Autodesk Inventor part; units mm, degrees
ref_plane "YZ Plane" through (0, 0, 0) normal (1, 0, 0) x (0, 1, 0)
ref_plane "XZ Plane" through (0, 0, 0) normal (0, 1, 0) x (-1, 0, 0)
ref_plane "XY Plane" through (0, 0, 0) normal (0, 0, 1) x (1, 0, 0)
sketch "Эскиз1" plane through (0, 0, 0) normal (0, 1, 0) x (-1, 0, 0)
  circle A0 centre (0, 0) radius 1.6
  dimension "d0" = 3.2
extrude "Выдавливание1" add sketch "Эскиз1" along normal blind 75
sketch "Эскиз2" plane through (0, 75, 0) normal (0, 1, 0) x (1, 0, 0)
  circle A0 centre (0, 0) radius 2.5
  dimension "d3" = 5
extrude "Выдавливание2" add sketch "Эскиз2" against normal blind 1
fillet "Сопряжение1" radius 1 1 edges at (-2.5, 74, 0)
sketch "Эскиз3" plane through (0, 0, 0) normal (0, -1, 0) x (1, 0, 0)
  circle A0 centre (0, 0) radius 2.5
extrude "Выдавливание3" add sketch "Эскиз3" against normal blind 1
fillet "Сопряжение2" radius 1 1 edges at (-2.5, 1, 0)
ref_plane "РабПлоскость1" through (-4.5, 3.005, 18.077) normal (-1, 0, 0) x (0, 0, -1)
sketch "Эскиз4" plane through (-4.5, 3.005, 18.077) normal (-1, 0, 0) x (0, 0, -1)
  line L0 (15.577, -71.995) -> (20.577, -71.995)
  line L1 (20.577, 3.005) -> (15.577, 3.005)
  point P0 (18.077, 3.005)
  dimension "d10" = 75
properties part number "vint"
Model file for the job. Use its own axes, mm. Give positions to 0.01 mm unless a question says otherwise; leave off trailing zeros. Loops run counter-clockwise (first coordinate to the right, second up) from the corner with the lowest first, then second, coordinate; pieces in that order, holes last.
Item 1: Slice it at B-B (z = 0). Write the cut outline in (x, y), plus the area to 3 significant figures.
Check values:
outline: (-2.5, 0) - (2.5, 0) arc R1 ccw to (1.6, 0.99) - (1.6, 74.01) arc R1 ccw to (2.5, 75) - (-2.5, 75) arc R1 ccw to (-1.6, 74.01) - (-1.6, 0.99) arc R1 ccw to start
area: 243 mm2
Item 2: Slice it at A-A (x = 0). Write the cut outline in (y, z).
Check values:
outline: (0, -2.5) arc R1 ccw to (0.99, -1.6) - (74.01, -1.6) arc R1 ccw to (75, -2.5) - (75, 2.5) arc R1 ccw to (74.01, 1.6) - (0.99, 1.6) arc R1 ccw to (0, 2.5) - close
Item 3: Drop flat-ended pins along their axis: P1, Ø3, axis at x = -0.5, z = 1.5, coming from the -Y side; P2, Ø1, axis at y = 48, z = 1.5, coming from the +X side; P3, Ø3, axis at x = 1.5, y = 16.5, coming from the -Z side. Give the stop position or say it passes through.
Check values:
P1: stops at y = 0
P2: stops at x = 1.25
P3: stops at z = -1.6
Item 4: Drill centre lines: line 1 along Z through (x, y) = (0.1, 39); line 2 along Y through (x, z) = (-2.05, 0). Where is each one in solid material? Low to high.
Check values:
line 1: z = -1.6 to 1.6
line 2: y = 0 to 0.84, 74.16 to 75
Item 5: Slice it at C-C (y = 5). Write the cut outline in (x, z).
Check values:
outline: circle Ø3.2 at (0, 0)
Item 6: Mould opens along Y. For faces 1 (the face through (0, 0, 0)), 2 (the face through (1.27, 36.99, 0.97)), 3 (the face through (0, 75, 0)) say: +Y half, -Y half, draft (parallel to the pull), parting line (faces both ways), or undercut.
Check values:
face 1: -Y half
face 2: undercut
face 3: +Y half
